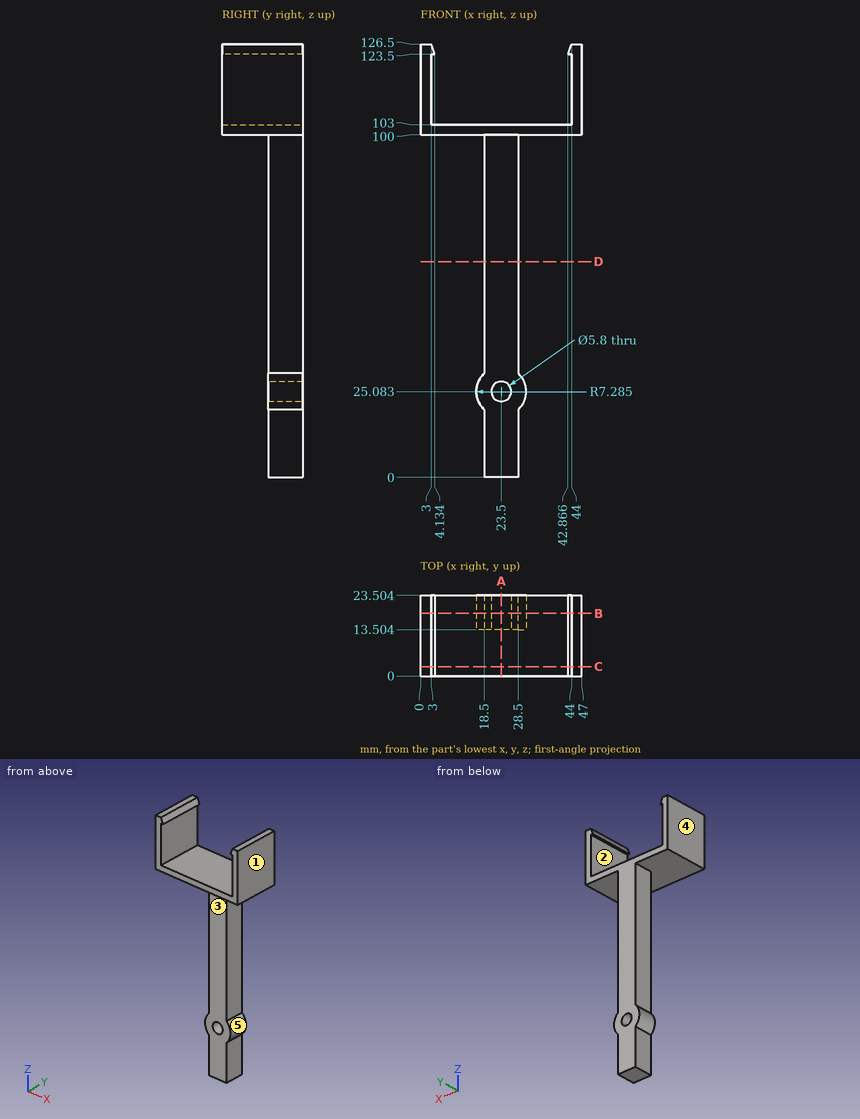
Source: three-view drawing plus pictorial views. Frame: mm from the lowest corner of the part. A direction names the side the tool comes from. Round coordinates to 2 decimals unless told otherwise and drop trailing zeros. Order: outer loops, then holes, each group sorted by start corner. A loop starts at its lowest first (then second) coordinate and runs counter-clockwise, first axis right, second up. Notation, with made-up numbers: (64, 23.25) - (84, 23.25) arc R26 ccw to (84, 48.25) - close; hole circle Ø10 at (-32.75, 35). An arc over 180 degrees is marked (long way). Write each question's results on one line, items separated by ' | '.
Item 1: First-contact query: pin 1 Ø7.5 at (x, z) = (23.5, 25.08) entering from -Y; pin 2 Ø7 at (x, y) = (14.5, 12) entering from -Z; pin 3 Ø3 at (y, z) = (18.5, 19.5) entering from -X. Flat tips, straight axial feed; report the tip coordinate or a pass-through.
Completed:
pin 1: y = 13.5 | pin 2: z = 20.73 | pin 3: x = 17.47
Item 2: Material intervals for line 1 along X through (y, z) = (3, 107); line 2 along Z through (x, y) = (10, 16.75); line 3 along X through (y, z) = (17.5, 50.5), sorted ascending. Write a range as [from, to].
Completed:
line 1: [0, 3], [44, 47] | line 2: [100, 103] | line 3: [18.5, 28.5]
Item 3: Section A-A, the plane x = 23.5. Return the cut outline in (y, z).
Completed:
outline: (0, 100) - (13.5, 100) - (13.5, 27.98) - (23.5, 27.98) - (23.5, 103) - (0, 103) - close; (13.5, 0) - (23.5, 0) - (23.5, 22.18) - (13.5, 22.18) - close
Item 4: Mould query, pull axis Z, two halves, no side actions, for the marked faces 4 and 5. Classes: pulls with the +Z half, pulls with the -Z half, needs draft (parallel to the pull), parting line crosses it, or undercut.
Completed:
face 4: needs draft | face 5: undercut
Item 5: Section B-B, the plane y = 18.25. Return the cut outline in (x, z) (1 decimal).
Completed:
outline: (0, 100) - (18.5, 100) - (18.5, 30.4) arc R7.3 ccw to (18.5, 19.8) - (18.5, 0) - (28.5, 0) - (28.5, 19.8) arc R7.3 ccw to (28.5, 30.4) - (28.5, 100) - (47, 100) - (47, 126.5) - (44, 126.5) - (42.9, 123.5) - (44, 123.5) - (44, 103) - (3, 103) - (3, 123.5) - (4.1, 123.5) - (3, 126.5) - (0, 126.5) - close; hole circle Ø5.8 at (23.5, 25.1)
Item 6: Reachability of the marked faces 1, 2 and 3 from +Z, -Z, +X, -X, +Y, -Y: full face, straight path, thin tool, end or side. Return the list, or none.
Completed:
face 1: +Z, -Z, +X, +Y, -Y | face 2: +Y, -Y | face 3: -Z, +X, -X, -Y
Item 7: Section D-D, the plane z = 63. Return the cut outline in (x, y), and give its area (3 significant figures).
Completed:
outline: (18.5, 13.5) - (28.5, 13.5) - (28.5, 23.5) - (18.5, 23.5) - close | area: 100 mm^2
Item 8: Section C-C, the plane y = 2.75. Return the cut outline in (x, z).
Completed:
outline: (0, 100) - (47, 100) - (47, 126.5) - (44, 126.5) - (42.87, 123.5) - (44, 123.5) - (44, 103) - (3, 103) - (3, 123.5) - (4.13, 123.5) - (3, 126.5) - (0, 126.5) - close
